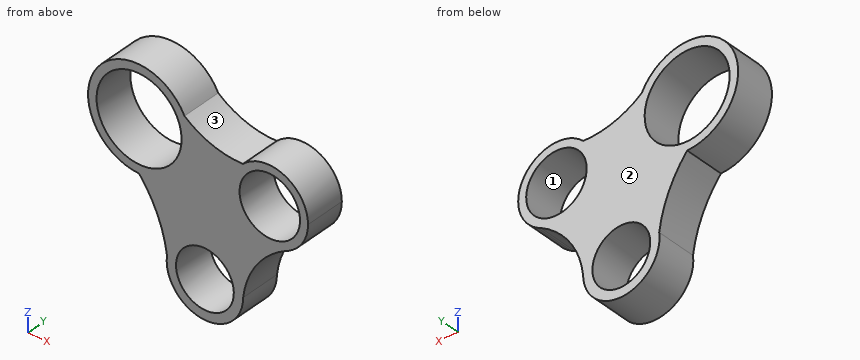
from build123d import *

# Parameters (mm, degrees)
SKETCH1_R           = 12.7
SKETCH1_R_2         = 10.587882435
SKETCH1_R_3         = 9.525
SKETCH1_R_4         = 7.199480632
SKETCH1_R_5         = 7.531788478
BOSS_EXTRUDE1_DEPTH = 10


with BuildPart() as part:
    # Sketch1 → Boss-Extrude1 (new body)
    # profile 1 of 4: a face of its own
    with BuildSketch(Plane(origin=(0, 0, 0), x_dir=(1, 0, 0), z_dir=(0, 1, 0))):
        with BuildLine():
            ThreePointArc((0, 12.7), (8.980256121, 8.980256121), (12.7, 0))
            ThreePointArc((12.7, 0), (12.349099919, -2.964748082), (11.315790364, -5.765664614))
            ThreePointArc((11.315790364, -5.765664614), (18.18064615, -2.153516868), (25.877180845, -1.185420811))
            ThreePointArc((25.877180845, -1.185420811), (24.696409251, 10.976736126), (36.457129285, 14.293021273))
            ThreePointArc((36.457129285, 14.293021273), (29.270833309, 20.788359993), (25.925837497, 29.879194827))
            ThreePointArc((25.925837497, 29.879194827), (17.031652126, 20.375106343), (6.959391743, 28.620335393))
            ThreePointArc((6.959391743, 28.620335393), (4.592983555, 20.173506773), (0, 12.7))
        make_face()
    # profile 2 of 4: a face of its own
    with BuildSketch(Plane(origin=(0, 0, 0), x_dir=(1, 0, 0), z_dir=(0, 1, 0))):
        Circle(SKETCH1_R)
        with Locations(Location((0, 0, 0), (0, 0, 270))):
            Circle(SKETCH1_R_2, mode=Mode.SUBTRACT)
    # profile 3 of 4: a face of its own
    with BuildSketch(Plane(origin=(0, 0, 0), x_dir=(1, 0, 0), z_dir=(0, 1, 0))):
        with Locations((16.400837497, 29.879194827)):
            Circle(SKETCH1_R_3)
        with Locations(Location((16.400837497, 29.879194827, 0), (0, 0, 270))):
            Circle(SKETCH1_R_4, mode=Mode.SUBTRACT)
    # profile 4 of 4: a face of its own
    with BuildSketch(Plane(origin=(0, 0, 0), x_dir=(1, 0, 0), z_dir=(0, 1, 0))):
        with BuildLine():
            ThreePointArc((36.457129285, 14.293021273), (24.696409251, 10.976736126), (25.877180845, -1.185420811))
            ThreePointArc((25.877180845, -1.185420811), (36.239101244, -3.183980484), (42.084961355, 5.601778145))
            ThreePointArc((42.084961355, 5.601778145), (40.798229992, 10.382631088), (37.285684743, 13.871794073))
            ThreePointArc((37.285684743, 13.871794073), (36.8689887, 14.077650841), (36.457129285, 14.293021273))
        make_face()
        with Locations(Location((32.559961355, 5.601778145, 0), (0, 0, 270))):
            Circle(SKETCH1_R_5, mode=Mode.SUBTRACT)
    extrude(amount=BOSS_EXTRUDE1_DEPTH)


solid = part.part
The listing builds one solid part. Answer for the finished solid, in the listing's coordinates (mm). Face numbers are marked on the shaded views. Give positions to 0.01 mm unless a question says otherwise; leave off trailing zeros. Loops run counter-clockwise (first coordinate to the right, second up) from the corner with the lowest first, then second, coordinate; pieces in that order, holes last. Notation, with made-up numbers: (39, 33.25) - (85, 33.25) arc R14 cw to (85, 54.25) - close; hole circle Ø2 at (-33.5, -37.75). An arc over 180 degrees is marked (long way). Answer as a JSON object with one key per item and string values.
1. A cutting plane is placed at A-A (z = -35). Write down the section's boundary in (x, y), then the cut area to 3 significant figures.
Determined:
{"outline": "(8.37, 0) - (11.34, 0) - (11.34, 10) - (8.37, 10) - close; (21.46, 0) - (24.43, 0) - (24.43, 10) - (21.46, 10) - close", "area": "59.4 mm²"}
2. A cutting plane is placed at C-C (y = 4.5). Write down the section's boundary in (x, z) (3 decimals).
Determined:
{"outline": "(0, -12.7) arc R31.666 cw to (6.959, -28.62) arc R9.525 ccw (long way) to (25.926, -29.879) arc R20.24 cw to (37.286, -13.872) arc R9.525 ccw (long way) to (25.877, 1.185) arc R21.71 cw to (11.316, 5.766) arc R12.7 ccw (long way) to start; hole circle Ø21.176 at (0, 0); hole circle Ø14.399 at (16.401, -29.879); hole circle Ø15.064 at (32.56, -5.602)"}
3. For a pull along Z with two mould halves and no side action, classify the marked faces 1, 2 and 3 as pulls with the +Z half, pulls with the -Z half, needs draft (parallel to the pull), parting line crosses it, or undercut.
Determined:
{"face 1": "undercut", "face 2": "needs draft", "face 3": "pulls with the +Z half"}
4. A cutting plane is placed at B-B (x = -7.5). Write down the section's boundary in (y, z).
Determined:
{"outline": "(0, -10.25) - (10, -10.25) - (10, -7.47) - (0, -7.47) - close; (0, 7.47) - (10, 7.47) - (10, 10.25) - (0, 10.25) - close"}
5. Flat-ended cylindrical pins translate along their axes: pin 1 Ø4 at (x, y) = (-1.5, 7) entering from -Z; pin 2 Ø3 at (y, z) = (1.5, -11.5) entering from +X; pin 3 Ø4 at (x, y) = (-7, 3) entering from +Z. Find the tip coordinate at first contact, or state that the pin passes through.
Determined:
{"pin 1": "z = -13.32", "pin 2": "x = 41.01", "pin 3": "z = 11.67"}
6. A cutting plane is placed at D-D (z = 0). Write down the section's boundary in (x, y).
Determined:
{"outline": "(-12.7, 0) - (-10.59, 0) - (-10.59, 10) - (-12.7, 10) - close; (10.59, 0) - (27.53, 0) - (27.53, 10) - (10.59, 10) - close; (37.59, 0) - (40.26, 0) - (40.26, 10) - (37.59, 10) - close"}
7. Find the intervals of material crossed by L1, parallel to X at y = 0.5, z = -1.5; L2, parallel to X at y = 7.75, z = -0.5; L3, parallel to Z at x = 19, y = 7, in increasing order. Write a range as [from, to].
Determined:
{"L1": "[-12.61, -10.48], [10.48, 26.24], [38.88, 41.16]", "L2": "[-12.69, -10.58], [10.58, 27.02], [38.1, 40.6]", "L3": "[-39.04, -36.59], [-23.17, 1.91]"}
